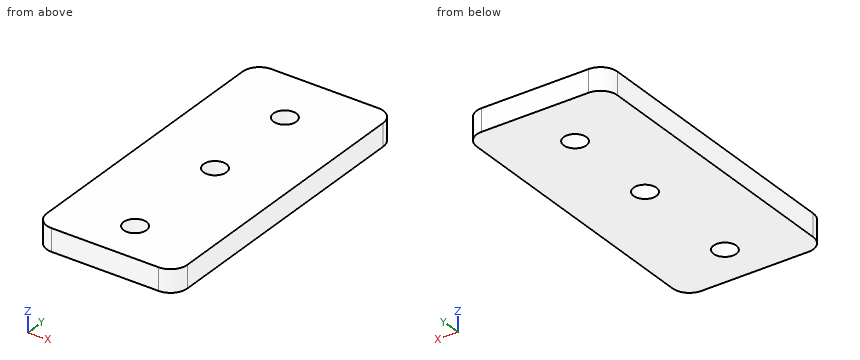
from build123d import *

# Parameters (mm, degrees)
SKETCH_1_W          = 25
SKETCH_1_H          = 55
EXTRUDE_1_DEPTH     = 2
SKETCH_2_R          = 2.025
CUT_EXTRUDE_1_DEPTH = 12
FILLET_1_R          = 3


with BuildPart() as part:
    # 草图1 → 凸台-拉伸1 (new body, symmetric)
    with BuildSketch(Plane.XY):
        Rectangle(SKETCH_1_W, SKETCH_1_H)
    extrude(amount=EXTRUDE_1_DEPTH, both=True)

    # 草图2 → 切除-拉伸1 (cut, symmetric)
    with BuildSketch(Plane.XY.offset(2)):
        with Locations((0, 17.5)):
            Circle(SKETCH_2_R)
        Circle(SKETCH_2_R)
        with Locations((0, -20)):
            Circle(SKETCH_2_R)
    extrude(amount=CUT_EXTRUDE_1_DEPTH, both=True, mode=Mode.SUBTRACT)

    # 圆角1
    fillet_1_edges = [part.edges().sort_by_distance(p)[0] for p in [
        (12.5, -27.5, 0),
        (-12.5, -27.5, 0),
        (-12.5, 27.5, 0),
        (12.5, 27.5, 0),
    ]]
    fillet(fillet_1_edges, radius=FILLET_1_R)


solid = part.part
CAD build for the part. Positions are in the model's coordinates, mm. Give positions to 0.01 mm unless a question says otherwise; leave off trailing zeros. Order: outer loops, then holes, each group sorted by start corner. A loop starts at its lowest first (then second) coordinate and runs counter-clockwise, first axis right, second up. Notation, with made-up numbers: (19.5, -36) - (43.5, -36) arc R33 ccw to (43.5, -5) - close; hole circle Ø2 at (-12, 55.25). An arc over 180 degrees is marked (long way). Write each question's results on one line, items separated by ' | '.
1. Saw through at D-D on y = -19. List the corners of the cut face in (x, z), and give its area (3 significant figures).
Calculated:
outline: (-12.5, -2) - (-1.76, -2) - (-1.76, 2) - (-12.5, 2) - close; (1.76, -2) - (12.5, -2) - (12.5, 2) - (1.76, 2) - close | area: 85.9 mm2
2. Probe L1, parallel to Y at x = 0, z = -0.1 (3 decimals); L2, parallel to Y at x = 0.75, z = 1.7; L3, parallel to X at y = 1.5, z = 1.6. List the from-to ranges inside material, lowest first. Write a range as from..to.
Calculated:
L1: y = -27.5..-22.025, -17.975..-2.025, 2.025..15.475, 19.525..27.5 | L2: y = -27.5..-21.88, -18.12..-1.88, 1.88..15.62, 19.38..27.5 | L3: x = -12.5..-1.36, 1.36..12.5
3. Saw through at C-C on z = 1.25. List the corners of the cut face in (x, y) (3 decimals).
Calculated:
outline: (-12.5, -24.5) arc R3 ccw to (-9.5, -27.5) - (9.5, -27.5) arc R3 ccw to (12.5, -24.5) - (12.5, 24.5) arc R3 ccw to (9.5, 27.5) - (-9.5, 27.5) arc R3 ccw to (-12.5, 24.5) - close; hole circle Ø4.05 at (0, -20); hole circle Ø4.05 at (0, 0); hole circle Ø4.05 at (0, 17.5)
4. Saw through at A-A on y = 0. List the corners of the cut face in (x, z) (3 decimals), and give its area (3 significant figures).
Calculated:
outline: (-12.5, -2) - (-2.025, -2) - (-2.025, 2) - (-12.5, 2) - close; (2.025, -2) - (12.5, -2) - (12.5, 2) - (2.025, 2) - close | area: 83.8 mm2
5. Pin check, flat tip, straight feed: pin 1 (6.5 mm diameter, centred on x = 0, y = 17.5, fed in from -Z). Stop position of the tip, or through.
Calculated:
pin 1: stops at z = -2
6. Saw through at B-B on x = 0. List the corners of the cut face in (y, z) (3 decimals).
Calculated:
outline: (-27.5, -2) - (-22.025, -2) - (-22.025, 2) - (-27.5, 2) - close; (-17.975, -2) - (-2.025, -2) - (-2.025, 2) - (-17.975, 2) - close; (2.025, -2) - (15.475, -2) - (15.475, 2) - (2.025, 2) - close; (19.525, -2) - (27.5, -2) - (27.5, 2) - (19.525, 2) - close
